```python
from build123d import *

# Parameters (mm, degrees)
SKETCH_2_R      = 1.6
EXTRUDE_1_DEPTH = 4
FILLET_1_R      = 5


with BuildPart() as part:
    # 草图2 → 凸台-拉伸1 (new body)
    with BuildSketch(Plane.XY):
        Polygon((0, 0), (40, 0), (40, 70), (120, 70), (120, 450), (40, 450), (0, 450), align=None)
        with Locations((20, 8)):
            Circle(SKETCH_2_R, mode=Mode.SUBTRACT)
        with Locations((20, 22)):
            Circle(SKETCH_2_R, mode=Mode.SUBTRACT)
        with Locations((27, 15)):
            Circle(SKETCH_2_R, mode=Mode.SUBTRACT)
        with Locations((13, 15)):
            Circle(SKETCH_2_R, mode=Mode.SUBTRACT)
        with Locations((20, 15)):
            Circle(SKETCH_2_R, mode=Mode.SUBTRACT)
        with Locations((115, 441)):
            Circle(SKETCH_2_R, mode=Mode.SUBTRACT)
        with Locations((5, 441)):
            Circle(SKETCH_2_R, mode=Mode.SUBTRACT)
    extrude(amount=EXTRUDE_1_DEPTH)

    # 圆角1
    fillet_1_edges = [part.edges().sort_by_distance(p)[0] for p in [
        (0, 450, 2),
        (120, 450, 2),
        (120, 70, 2),
        (40, 70, 2),
        (40, 0, 2),
        (0, 0, 2),
    ]]
    fillet(fillet_1_edges, radius=FILLET_1_R)


solid = part.part
```
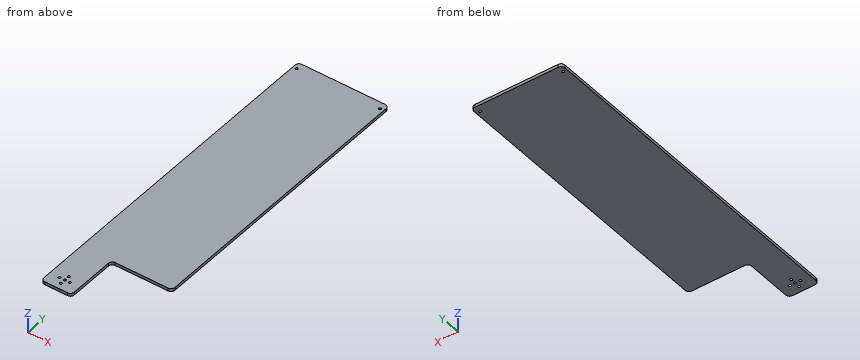
Work out the finished part from the listing and answer in its coordinate system (mm). Give positions to 0.01 mm unless a question says otherwise; leave off trailing zeros. Write each loop counter-clockwise with the first axis right and the second up, starting at its lowest first coordinate (ties: lowest second). Pieces come first, ordered by that corner, then holes. Notation, with made-up numbers: (82, 4) -> (87, 4) arc R12 ccw to (87, 25) -> close; hole circle Ø4 at (-14, 4). An arc over 180 degrees is marked (long way). Write item = value, one per line.
Q1. Flat-ended cylindrical pins translate along their axes: pin 1 Ø3.5 at (x, y) = (20, 15) entering from -Z; pin 2 Ø2.5 at (x, y) = (20, 22) entering from +Z; pin 3 Ø1.2 at (y, z) = (32.5, 3) entering from +X. Find the tip coordinate at first contact, or state that the pin passes through.
Computed values:
pin_1 = 0
pin_2 = through
pin_3 = 40
Q2. Section B-B on y = 40 is taken. Determine the outline of the cut face in (x, z), and give its area (3 significant figures).
Computed values:
outline = (0, 0) -> (40, 0) -> (40, 4) -> (0, 4) -> close
area = 160 mm^2
Q3. Section C-C on x = 91 is taken. Determine the outline of the cut face in (y, z), and give its area (3 significant figures).
Computed values:
outline = (70, 0) -> (450, 0) -> (450, 4) -> (70, 4) -> close
area = 1,520 mm^2
Q4. Section A-A on z = 1.9 is taken. Determine the outline of the cut face in (x, y), and give its area (3 significant figures).
Computed values:
outline = (0, 5) arc R5 ccw to (5, 0) -> (35, 0) arc R5 ccw to (40, 5) -> (40, 65) arc R5 cw to (45, 70) -> (115, 70) arc R5 ccw to (120, 75) -> (120, 445) arc R5 ccw to (115, 450) -> (5, 450) arc R5 ccw to (0, 445) -> close; hole circle Ø3.2 at (5, 441); hole circle Ø3.2 at (13, 15); hole circle Ø3.2 at (20, 8); hole circle Ø3.2 at (20, 15); hole circle Ø3.2 at (20, 22); hole circle Ø3.2 at (27, 15); hole circle Ø3.2 at (115, 441)
area = 48,300 mm^2
Q5. Consider line 1 along Y through (x, z) = (20, 1); line 2 along X through (y, z) = (441, 3.1); line 3 along X through (y, z) = (50, 2.75). Determine where each line is inside the solid, lowest interval first.
Computed values:
line_1 = 0 to 6.4, 9.6 to 13.4, 16.6 to 20.4, 23.6 to 450
line_2 = 0 to 3.4, 6.6 to 113.4, 116.6 to 120
line_3 = 0 to 40
